Can you work these out from the model? Positions are in its coordinate system, mm. A direction names the side the tool comes from. Round coordinates to 2 decimals unless told otherwise and drop trailing zeros. Loops run counter-clockwise (first coordinate to the right, second up) from the corner with the lowest first, then second, coordinate; pieces in that order, holes last.
(1) Which directions (+Z, -Z, +X, -X, +Y, -Y) give clear straight access to the entire face, cutting with the end or side of a thin tool? Please do faces 4 (the face through (5.12, 3.22, 5.39)), 5 (the face through (5, 6.35, 7)).
(2) I want a section at B-B on z = -5.9. Write out the boundary of the cut face in (x, y) (3 decimals).
(3) Thinking about a two-plate mould opening in X: for faces 1 (the face through (-9, 7.95, 0)), 2 (the face through (-10.55, 4, 0)), 3 (the face through (-2.586, 3.219, -7.333)), which applies, released by +X, released by -X, zero draft, split by the parting line, or undercut?
(4) Will this pin go through, and if not, where does the flat tip stop? pin 1 Ø7.5 at (x, z) = (0.5, 3) entering from +Y.
(5) I want a section at A-A on y = 4. Write out the boundary of the cut face in (x, z) (3 decimals).
(6) I want a section at D-D on x = -4.5. Write out the boundary of the cut face in (y, z) (3 decimals).
(7) If I drill on line 1 along Z through (x, y) = (-3.5, 4.75) (3 decimals); line 2 along X through (y, z) = (4.25, -5.9) (3 decimals); line 3 along Z through (x, y) = (3.5, 4.75) (3 decimals), over which ranges is the centre line in solid material (lowest first)?
(8) I want a section at C-C on y = 1.5. Write out the boundary of the cut face in (x, z) (3 decimals), plus the area to 3 significant figures.
Autodesk Inventor part; units mm, degrees
ref_plane "YZ Plane" through (0, 0, 0) normal (1, 0, 0) x (0, 1, 0)
ref_plane "XZ Plane" through (0, 0, 0) normal (0, 1, 0) x (-1, 0, 0)
ref_plane "XY Plane" through (0, 0, 0) normal (0, 0, 1) x (1, 0, 0)
sketch "Sketch1" plane through (0, 0, 0) normal (0, 1, 0) x (-1, 0, 0)
  line L0 (-10.55, -13.05) -> (10.55, -13.05)
  line L1 (10.55, -13.05) -> (10.55, 13.05)
  line L2 (10.55, 13.05) -> (-10.55, 13.05)
  line L3 (-10.55, 13.05) -> (-10.55, -13.05)
  line L4 (-10.55, -13.05) -> (10.55, 13.05) construction
  line L5 (10.55, -13.05) -> (-10.55, 13.05) construction
  point P0 (0, 0)
  dimension "d0" = 26.1
  dimension "d1" = 21.1
extrude "Extrusion1" add sketch "Sketch1" along normal blind 7.95
sketch "Sketch2" plane through (0, 7.95, 0) normal (0, 1, 0) x (1, 0, 0)
  line L0 (7.375, -9.875) -> (-7.375, -9.875)
  line L1 (-7.375, -9.875) -> (-7.375, 9.875)
  line L2 (-7.375, 9.875) -> (7.375, 9.875)
  line L3 (7.375, 9.875) -> (7.375, -9.875)
  line L4 (7.375, -9.875) -> (-7.375, 9.875) construction
  line L5 (-7.375, -9.875) -> (7.375, 9.875) construction
  point P0 (0, 0)
  dimension "d4" = 19.75
  dimension "d5" = 14.75
extrude "Extrusion2" cut sketch "Sketch2" against normal blind 4.775
sketch "Sketch3" plane through (0, 3.175, 0) normal (0, 1, 0) x (1, 0, 0)
  circle A0 centre (-3.5, 5.9) radius 3
  circle A1 centre (3.5, -5.9) radius 3
  point P0 (0, 0)
  dimension "d8" = 11.8
  dimension "d9" = 7
  dimension "d10" = 5.9
  dimension "d11" = 3.5
  dimension "d12" = 6
  dimension "d13" = 6
extrude "Extrusion3" add sketch "Sketch3" along normal blind 3.175
sketch "Sketch4" plane through (3.5, 6.35, 5.9) normal (0, 1, 0) x (1, 0, 0)
  circle A0 centre (0, 0) radius 1.7
  circle A1 centre (-7, 11.8) radius 3
  circle A2 centre (-7, 11.8) radius 1.7
  point P0 (-3.5, 5.9)
  dimension "d16" = 3.4
  dimension "d17" = 3.4
extrude "Extrusion4" cut sketch "Sketch4" against normal through all contours A0 | A2
fillet "Fillet1" radius 3.175 4 edges at (10.55, 3.975, 13.05) (10.55, 3.975, -13.05) (-10.55, 3.975, 13.05) (-10.55, 3.975, -13.05)
equation "\"d13\" = d12"
equation "\"d16\" = m3_clearance"
equation "\"d17\" = m3_clearance"
equation "\"m3_heat_set_insert\" = 4"
equation "\"m3_clearance\" = 3.4"
equation "\"m3_heat_set_depth\" = 7"
equation "\"robot_diameter\" = 354"
equation "\"hardboard_thickness\" = 5"
equation "\"motor_centerline_height\" = 13"
properties part number "environmental_sensor_case"
Filled sheet:
1. face 4: +Y, -Y
1. face 5: +Y
2. outline: (-10.55, 0) - (-5.2, 0) - (-5.2, 6.35) - (-6.5, 6.35) - (-6.5, 3.175) - (-7.375, 3.175) - (-7.375, 7.95) - (-10.55, 7.95) - close; (-1.8, 0) - (10.55, 0) - (10.55, 7.95) - (7.375, 7.95) - (7.375, 3.175) - (-0.5, 3.175) - (-0.5, 6.35) - (-1.8, 6.35) - close
3. face 1: zero draft
3. face 2: released by -X
3. face 3: undercut
4. pin 1: stops at y = 6.35
5. outline: (-10.55, -9.875) arc R3.175 ccw to (-7.375, -13.05) - (7.375, -13.05) arc R3.175 ccw to (10.55, -9.875) - (10.55, 9.875) arc R3.175 ccw to (7.375, 13.05) - (-7.375, 13.05) arc R3.175 ccw to (-10.55, 9.875) - close; circle Ø6 at (-3.5, -5.9); circle Ø6 at (3.5, 5.9); hole (-7.375, -9.875) - (7.375, -9.875) - (7.375, 9.875) - (-7.375, 9.875) - close; hole circle Ø3.4 at (-3.5, -5.9); hole circle Ø3.4 at (3.5, 5.9)
6. outline: (0, -13.05) - (7.95, -13.05) - (7.95, -9.875) - (3.175, -9.875) - (3.175, -8.728) - (6.35, -8.728) - (6.35, -7.275) - (0, -7.275) - close; (0, -4.525) - (6.35, -4.525) - (6.35, -3.072) - (3.175, -3.072) - (3.175, 9.875) - (7.95, 9.875) - (7.95, 13.05) - (0, 13.05) - close
7. line 1: z = -13.05 to -9.875, -8.9 to -7.6, -4.2 to -2.9, 9.875 to 13.05
7. line 2: x = -10.55 to -7.375, -6.5 to -5.2, -1.8 to -0.5, 7.375 to 10.55
7. line 3: z = -13.05 to -9.875, 2.9 to 4.2, 7.6 to 8.9, 9.875 to 13.05
8. outline: (-10.55, -9.875) arc R3.175 ccw to (-7.375, -13.05) - (7.375, -13.05) arc R3.175 ccw to (10.55, -9.875) - (10.55, 9.875) arc R3.175 ccw to (7.375, 13.05) - (-7.375, 13.05) arc R3.175 ccw to (-10.55, 9.875) - close; hole circle Ø3.4 at (-3.5, -5.9); hole circle Ø3.4 at (3.5, 5.9)
8. area: 524 mm2
